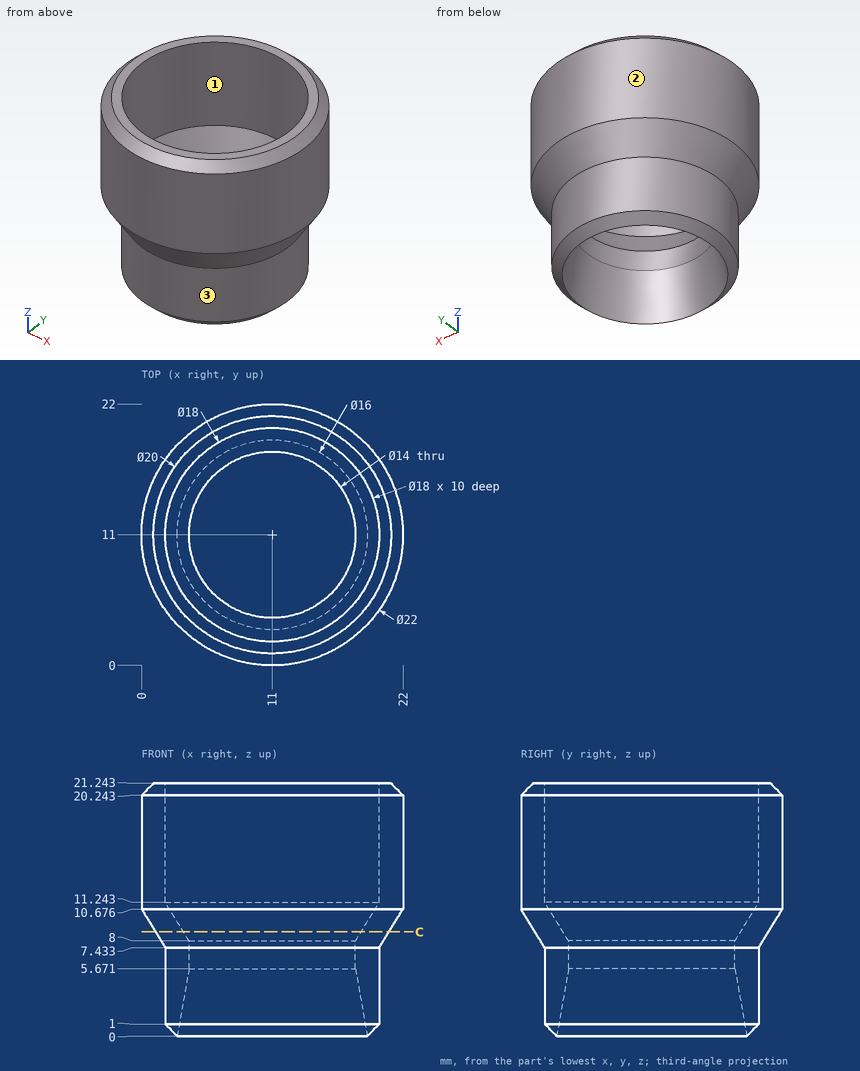
Part print with two shaded views. Sizes in mm from the minimum x, y, z corner. A direction names the side the tool comes from. Round coordinates to 2 decimals unless told otherwise and drop trailing zeros. Order: outer loops, then holes, each group sorted by start corner. A loop starts at its lowest first (then second) coordinate and runs counter-clockwise, first axis right, second up. Notation, with made-up numbers: M 35.25,84.25 L 91.25,84.25 A9 ccw 91.25,95.25 Z; hole C -16,72 d7. An arc over 180 degrees is marked long. Use CSV: the item, a comma, the result in double quotes. Start each with the question number.
(1) Flat gauge pins, fed straight in: P1, Ø3, axis at x = 4.5, z = 9.5, coming from the +Y side; P2, Ø8, axis at x = 17.5, z = 8, coming from the +Y side; P3, Ø1.5, axis at x = 9, z = 14, coming from the +Y side; P4, Ø12.5, axis at x = 11, y = 11, coming from the -Z side. Where does each tip first touch, or does it go through?
(2) Tool access for the marked faces 1, 2 and 3: list every direction of +Z, -Z, +X, -X, +Y, -Y with a clear straight run to the whole face (end or side of a thin tool).
(3) Drill centre lines: probe 1 along Y at (x, z) = (11, 13.5); probe 2 along Y at (x, z) = (11, 7.2). Where is each one in solid material? Low to high.
(4) Cut at C-C on z = 8.75. List the corners of the cut face in (x, y) (1 decimal).
Findings:
1,P1,"stops at y = 20.49"
1,P2,"stops at y = 21.42"
1,P3,"stops at y = 21.93"
1,P4,"passes through"
2,face 1,"+Z"
2,face 2,"+Z, -Z"
2,face 3,"-Z"
3,probe 1,"y = 0 to 2, 20 to 22"
3,probe 2,"y = 2 to 4, 18 to 20"
4,outline,"C 11,11 d19.6; hole C 11,11 d14.9"
